Build history of the part. All positions in model axes, mm. A direction names the side the tool comes from. Round coordinates to 2 decimals unless told otherwise and drop trailing zeros. Order: outer loops, then holes, each group sorted by start corner. A loop starts at its lowest first (then second) coordinate and runs counter-clockwise, first axis right, second up. Notation, with made-up numbers: (18, 17) - (22, 17) arc R17 ccw to (22, 35) - close; hole circle Ø5 at (75.25, 16.5). An arc over 180 degrees is marked (long way). One line per question, with ' | ' between items. Start each with the question number.
Autodesk Inventor part; units mm, degrees
ref_plane "YZ Plane" through (0, 0, 0) normal (1, 0, 0) x (0, 1, 0)
ref_plane "XZ Plane" through (0, 0, 0) normal (0, 1, 0) x (-1, 0, 0)
ref_plane "XY Plane" through (0, 0, 0) normal (0, 0, 1) x (1, 0, 0)
sketch "Sketch1" plane through (0, 0, 0) normal (0, 1, 0) x (-1, 0, 0)
  point P0 (0, 0)
sketch "Sketch2" plane through (0, 0, 0) normal (1, 0, 0) x (0, 1, 0)
  line L0 (1.9877, 1.8129) -> (-22.0123, 1.8129)
  line L1 (-22.0123, 1.8129) -> (-22.0123, -22.1871)
  line L2 (-22.0123, -22.1871) -> (1.9877, -22.1871)
  line L3 (1.9877, -22.1871) -> (1.9877, 1.8129)
  point P0 (0, 0)
extrude "Extrusion1" add sketch "Sketch2" along normal blind 20
sketch "Sketch3" plane through (20, 0, 0) normal (1, 0, 0) x (0, 0, -1)
  circle A0 centre (10.1871, -10.0123) radius 10
  line L0 (22.1871, 1.9877) -> (-1.8129, 1.9877)
  line L1 (-1.8129, 1.9877) -> (-1.8129, -22.0123)
  point P0 (0, 0)
extrude "Extrusion2" add sketch "Sketch3" along normal blind 10
sketch "Sketch4" plane through (30, -10.0123, -10.1871) normal (1, 0, 0) x (0, 0, -1)
  circle A0 centre (0, 0) radius 3
  point P0 (-10.1871, 10.0123)
extrude "Extrusion3" add sketch "Sketch4" along normal blind 10
chamfer "Chamfer1" distance 1 angle 45 13 edges at (0, 1.9877, -10.1871) (10, 1.9877, -22.1871) (20, 1.9877, -10.1871) (10, 1.9877, 1.8129) (20, -10.0123, 1.8129) (20, -10.0123, -22.1871) (30, -10.0123, -0.1871) (40, -10.0123, -7.1871) (0, -10.0123, 1.8129) (10, -22.0123, 1.8129) (20, -22.0123, -10.1871) (0, -10.0123, -22.1871) (0, -22.0123, -10.1871)
sketch "Sketch5" plane through (1, 1.9877, 0.8129) normal (0, 1, 0) x (1, 0, 0)
  point P0 (-1, 0.8129)
properties part number "motor(1 shaft)" material "Steel, Alloy"
Item 1: Pin check, flat tips, straight feed: pin 1 (8 mm diameter, centred on x = 30.5, z = -18, fed in from -Y); pin 2 (1 mm diameter, centred on y = -2, z = -9, fed in from +X); pin 3 (3 mm diameter, centred on x = 35, z = -7.5, fed in from -Y). Stop position of each tip, or through.
Item 2: 3-axis set-ups, long thin cutter, end or side, ignore diameter. For faces 1 (the face through (30, -10, -14)), 2 (the face through (19.507, -10.351, -21.68)): which of +Z, -Z, +X, -X, +Y, -Y reach the whole face in a straight line?
Item 3: Slice it at B-B (x = 37.5). Write the cut outline in (y, z), plus the area to 3 significant figures.
Item 4: Wall check: line 1 along X through (y, z) = (-10.75, -13.5); line 2 along X through (y, z) = (-18.5, -17.5); line 3 along Y through (x, z) = (28, -9.75). Give the ranges that are in metal, low to high. Write a range as [from, to].
Item 5: Slice it at A-A (x = 24). Write the cut outline in (y, z).
A:
1) pin 1: y = -19.13 | pin 2: x = 30 | pin 3: y = -12.77
2) face 1: +X | face 2: -Z, +X, +Y, -Y
3) outline: circle Ø6 at (-10.01, -10.19) | area: 28.3 mm^2
4) line 1: [0, 30] | line 2: [0, 20] | line 3: [-20, -0.02]
5) outline: circle Ø20 at (-10.01, -10.19)
